Input: part model. Units: mm. Frame: model coordinates. A direction names the side the tool comes from. Round coordinates to 2 decimals unless told otherwise and drop trailing zeros. Loops run counter-clockwise (first coordinate to the right, second up) from the corner with the lowest first, then second, coordinate; pieces in that order, holes last. Notation, with made-up numbers: (-12, 25.5) -> (8, 25.5) arc R13 cw to (8, 47.5) -> close; hole circle Ø11 at (0.25, 70). An arc over 180 degrees is marked (long way). Answer as a JSON object with one key per item and string values. Group by question number.
Item 1: Section query C-C on x = 5.5. Return loops of the section in (y, z).
Item 2: Set-up query: faces 5 (the flat face through (-12, 17, 4)), 6 (the flat face through (2, -27, -2)), 7 (the flat face through (9.5, -32, 4)), 8 (the flat face through (2.7, -23, -3.5)). Return all of +Z, -Z, +X, -X, +Y, -Y with unobstructed straight access to the full face (end or side cutting, diameter ignored); none if empty.
Item 3: Section query A-A on y = 6. Return loops of the section in (x, z).
Item 4: Section query B-B on z = 11.2. Return loops of the section in (x, y).
Item 5: Pin query (flat end, axial travel): pin 1 (15.5 mm diameter, centred on x = 7.5, y = -9.5, fed in from -Z); pin 2 (7.5 mm diameter, centred on x = -5, z = 7, fed in from +Y); pin 3 (0.5 mm diameter, centred on x = -2.5, z = 1, fed in from -Y); pin 4 (3 mm diameter, centred on x = -8, z = 11.2, fed in from +Y). Return the tip coordinate at first contact, or that it passes through.
Item 6: Section query D-D on x = 10.5. Return loops of the section in (y, z).
Item 7: Draft query along Z for faces 1 (the flat face through (3, -30, 9)), 2 (the flat face through (3, -24, -4)), 3 (the flat face through (-14, -17, 7)), 4 (the flat face through (-11, 15, 7)). Return one class per face: released by +Z, released by -Z, zero draft, split by the parting line, or undercut.
Item 8: Material intervals for line 1 (Y direction, x = -10, z = 5.75); line 2 (X direction, y = 15.05, z = 4.5); line 3 (Z direction, x = 13, y = -31.2), sorted ascending. Write a range as [from, to].
from build123d import *

# Parameters (mm, degrees)
SKETCH_1_W           = 35
SKETCH_1_H           = 53
EXTRUDE_1_DEPTH      = 2
SKETCH_2_W           = 2
SKETCH_2_H           = 53
EXTRUDE_2_DEPTH      = 13.2
SKETCH_3_W           = 31
SKETCH_3_H           = 3
EXTRUDE_3_DEPTH      = 7.2
SKETCH_4_W           = 31
SKETCH_4_H           = 3
EXTRUDE_4_DEPTH      = 13.2
CUT_EXTRUDE_1_REACH  = 57.956
SKETCH_5_R           = 1.25
SKETCH_7_W           = 31
SKETCH_7_H           = 3
CUT_EXTRUDE_2_DEPTH  = 2.2
SKETCH_8_W           = 31
SKETCH_8_H           = 3
CUT_EXTRUDE_3_DEPTH  = 2
SKETCH_10_W          = 11
SKETCH_10_H          = 3
CUT_EXTRUDE_4_DEPTH  = 4
CUT_EXTRUDE_START    = -3
SKETCH_9_R           = 1.25
CUT_EXTRUDE_5_DEPTH  = 3
SKETCH_14_W          = 31
SKETCH_14_H          = 3
CUT_EXTRUDE_8_DEPTH  = 5
SKETCH_15_W          = 35
SKETCH_15_H          = 53
SKETCH_15_W_2        = 26
SKETCH_15_H_2        = 36
EXTRUDE_5_DEPTH      = 1
SKETCH_15_3_W        = 26
SKETCH_15_3_H        = 36
CUT_EXTRUDE_9_DEPTH  = 2
SKETCH_15_4_W        = 35
SKETCH_15_4_H        = 53
SKETCH_15_4_W_2      = 26
SKETCH_15_4_H_2      = 36
EXTRUDE_6_DEPTH      = 1
SKETCH_14_2_W        = 31
SKETCH_14_2_H        = 3
CUT_EXTRUDE_10_DEPTH = 7.2
SKETCH_21_W          = 31
SKETCH_21_H          = 3
CUT_EXTRUDE_11_DEPTH = 4
SKETCH_9_6_W         = 31
SKETCH_9_6_H         = 4
SKETCH_9_6_R         = 1.25
EXTRUDE_8_DEPTH      = 3
SKETCH_9_7_W         = 31
SKETCH_9_7_H         = 4
SKETCH_9_7_R         = 1.25
CUT_EXTRUDE_12_DEPTH = 3
SKETCH_23_W          = 31
SKETCH_23_H          = 3
EXTRUDE_9_DEPTH      = 2
SKETCH_24_W          = 31
SKETCH_24_H          = 3
CUT_EXTRUDE_13_DEPTH = 7.2
SKETCH_25_R          = 1.2
CUT_EXTRUDE_14_DEPTH = 3
SKETCH_15_5_W        = 35
SKETCH_15_5_H        = 53
SKETCH_15_5_W_2      = 26
SKETCH_15_5_H_2      = 36
EXTRUDE_10_DEPTH     = 2
SKETCH_28_W          = 31
SKETCH_28_H          = 2.1
CUT_EXTRUDE_15_DEPTH = 47
SKETCH_21_2_W        = 31
SKETCH_21_2_H        = 3
CUT_EXTRUDE_16_DEPTH = 6
SKETCH_12_W          = 2
SKETCH_12_H          = 10
CUT_EXTRUDE_17_DEPTH = 13.2
SKETCH_12_2_W        = 2
SKETCH_12_2_H        = 10
EXTRUDE_11_DEPTH     = 8.2
SKETCH_33_W          = 14
SKETCH_33_H          = 5
CUT_EXTRUDE_18_DEPTH = 3
SKETCH_34_W          = 21
SKETCH_34_H          = 3
CUT_EXTRUDE_19_DEPTH = 5
CUT_EXTRUDE_20_DEPTH = 0.1
CUT_EXTRUDE_21_DEPTH = 0.1
SKETCH_38_W          = 31
SKETCH_38_H          = 47
SKETCH_38_W_2        = 26
SKETCH_38_H_2        = 36
EXTRUDE_12_DEPTH     = 2
SKETCH_39_W          = 26
SKETCH_39_H          = 36
CUT_EXTRUDE_22_DEPTH = 2
SKETCH_40_W          = 35
SKETCH_40_H          = 53
SKETCH_40_W_2        = 26
SKETCH_40_H_2        = 36
EXTRUDE_13_DEPTH     = 2
SKETCH_41_W          = 31
SKETCH_41_H          = 47
SKETCH_41_W_2        = 26
SKETCH_41_H_2        = 36
CUT_EXTRUDE_23_DEPTH = 2
EXTRUDE_14_DEPTH     = 1.8


with BuildPart() as part:
    # 草图1 → 凸台-拉伸1 (new body)
    with BuildSketch(Plane.XY):
        with Locations((2.5, -6.5)):
            Rectangle(SKETCH_1_W, SKETCH_1_H)
    extrude(amount=EXTRUDE_1_DEPTH)

    # 草图2 → 凸台-拉伸2 (add)
    with BuildSketch(Plane.XY.offset(2)):
        with Locations((-14, -6.5)):
            Rectangle(SKETCH_2_W, SKETCH_2_H)
        with Locations((19, -6.5)):
            Rectangle(SKETCH_2_W, SKETCH_2_H)
    extrude(amount=EXTRUDE_2_DEPTH)

    # 草图3 → 凸台-拉伸3 (add)
    with BuildSketch(Plane.XY.offset(2)):
        with Locations((2.5, 18.5)):
            Rectangle(SKETCH_3_W, SKETCH_3_H)
        with Locations((2.5, -31.5)):
            Rectangle(SKETCH_3_W, SKETCH_3_H)
    extrude(amount=EXTRUDE_3_DEPTH)

    # 草图4 → 凸台-拉伸4 (add)
    with BuildSketch(Plane.XY.offset(2)):
        with Locations((2.5, 15.5)):
            Rectangle(SKETCH_4_W, SKETCH_4_H)
        with Locations((2.5, -28.5)):
            Rectangle(SKETCH_4_W, SKETCH_4_H)
    extrude(amount=EXTRUDE_4_DEPTH)

    # 草图5 → 切除-拉伸1 (cut, up to next)
    with BuildSketch(Plane(origin=(0, 17, 0), x_dir=(1, 0, 0), z_dir=(0, 1, 0)), mode=Mode.PRIVATE) as cut_extrude_1_sk1:
        with Locations(Location((-8, -11.2, 0), (0, 0, 270))):
            Circle(SKETCH_5_R)
    cut_extrude_1_tool1 = extrude(cut_extrude_1_sk1.sketch, amount=-CUT_EXTRUDE_1_REACH, mode=Mode.PRIVATE) & part.part
    # 草图5 → 切除-拉伸1 (cut, up to next)
    with BuildSketch(Plane(origin=(0, 17, 0), x_dir=(1, 0, 0), z_dir=(0, 1, 0)), mode=Mode.PRIVATE) as cut_extrude_1_sk2:
        with Locations(Location((2.5, -11.2, 0), (0, 0, 270))):
            Circle(SKETCH_5_R)
    cut_extrude_1_tool2 = extrude(cut_extrude_1_sk2.sketch, amount=-CUT_EXTRUDE_1_REACH, mode=Mode.PRIVATE) & part.part
    # 草图5 → 切除-拉伸1 (cut, up to next)
    with BuildSketch(Plane(origin=(0, 17, 0), x_dir=(1, 0, 0), z_dir=(0, 1, 0)), mode=Mode.PRIVATE) as cut_extrude_1_sk3:
        with Locations(Location((13, -11.2, 0), (0, 0, 270))):
            Circle(SKETCH_5_R)
    cut_extrude_1_tool3 = extrude(cut_extrude_1_sk3.sketch, amount=-CUT_EXTRUDE_1_REACH, mode=Mode.PRIVATE) & part.part
    add(cut_extrude_1_tool1.solids().sort_by_distance((-8, 17, 11.2))[0], mode=Mode.SUBTRACT)
    add(cut_extrude_1_tool2.solids().sort_by_distance((2.5, 17, 11.2))[0], mode=Mode.SUBTRACT)
    add(cut_extrude_1_tool3.solids().sort_by_distance((13, 17, 11.2))[0], mode=Mode.SUBTRACT)

    # 草图7 → 切除-拉伸2 (cut)
    with BuildSketch(Plane.XY.offset(15.2)):
        with Locations((2.5, 15.5)):
            Rectangle(SKETCH_7_W, SKETCH_7_H)
    extrude(amount=-CUT_EXTRUDE_2_DEPTH, mode=Mode.SUBTRACT)

    # 草图8 → 切除-拉伸3 (cut)
    with BuildSketch(Plane.XY.offset(15.2)):
        with Locations((2.5, -28.5)):
            Rectangle(SKETCH_8_W, SKETCH_8_H)
    extrude(amount=-CUT_EXTRUDE_3_DEPTH, mode=Mode.SUBTRACT)

    # 草图10 → 切除-拉伸4 (cut)
    with BuildSketch(Plane.XY.offset(13.2)):
        with Locations((2.5, -28.5)):
            Rectangle(SKETCH_10_W, SKETCH_10_H)
    extrude(amount=-CUT_EXTRUDE_4_DEPTH, mode=Mode.SUBTRACT)

    # 草图9 → 切除-拉伸5 (cut)
    with BuildSketch(Plane.XZ.offset(30).offset(CUT_EXTRUDE_START)):
        with Locations(Location((-8, 11.2, 0), (0, 0, 90))):
            Circle(SKETCH_9_R)
        with Locations(Location((13, 11.2, 0), (0, 0, 90))):
            Circle(SKETCH_9_R)
    extrude(amount=CUT_EXTRUDE_5_DEPTH, mode=Mode.SUBTRACT)

    # 草图14 → 切除-拉伸8 (cut)
    with BuildSketch(Plane.XY.offset(9.2)):
        with Locations((2.5, 18.5)):
            Rectangle(SKETCH_14_W, SKETCH_14_H)
    extrude(amount=-CUT_EXTRUDE_8_DEPTH, mode=Mode.SUBTRACT)

    # 草图15 → 凸台-拉伸5 (add)
    with BuildSketch(Plane(origin=(0, 0, 0), x_dir=(-1, 0, 0), z_dir=(0, 0, -1))):
        with Locations((-2.5, -6.5)):
            Rectangle(SKETCH_15_W, SKETCH_15_H)
        with Locations((-2.5, -5)):
            Rectangle(SKETCH_15_W_2, SKETCH_15_H_2, mode=Mode.SUBTRACT)
    extrude(amount=EXTRUDE_5_DEPTH)

    # 草图15<3> → 切除-拉伸9 (cut)
    with BuildSketch(Plane(origin=(0, 0, 0), x_dir=(-1, 0, 0), z_dir=(0, 0, -1))):
        with Locations((-2.5, -5)):
            Rectangle(SKETCH_15_3_W, SKETCH_15_3_H)
    extrude(amount=-CUT_EXTRUDE_9_DEPTH, mode=Mode.SUBTRACT)

    # 草图15<4> → 凸台-拉伸6 (add)
    with BuildSketch(Plane(origin=(0, 0, 0), x_dir=(-1, 0, 0), z_dir=(0, 0, -1))):
        with Locations((-2.5, -6.5)):
            Rectangle(SKETCH_15_4_W, SKETCH_15_4_H)
        with Locations((-2.5, -5)):
            Rectangle(SKETCH_15_4_W_2, SKETCH_15_4_H_2, mode=Mode.SUBTRACT)
    extrude(amount=EXTRUDE_6_DEPTH)

    # 草图14<2> → 切除-拉伸10 (cut)
    with BuildSketch(Plane.XY.offset(9.2)):
        with Locations((2.5, 18.5)):
            Rectangle(SKETCH_14_2_W, SKETCH_14_2_H)
    extrude(amount=-CUT_EXTRUDE_10_DEPTH, mode=Mode.SUBTRACT)

    # 草图21 → 切除-拉伸11 (cut)
    with BuildSketch(Plane.XY.offset(13)):
        with Locations((2.5, 15.5)):
            Rectangle(SKETCH_21_W, SKETCH_21_H)
    extrude(amount=-CUT_EXTRUDE_11_DEPTH, mode=Mode.SUBTRACT)

    # 草图9<6> → 凸台-拉伸8 (add)
    with BuildSketch(Plane.XZ.offset(30)):
        with Locations((2.5, 11.2)):
            Rectangle(SKETCH_9_6_W, SKETCH_9_6_H)
        with Locations((13, 11.2)):
            Circle(SKETCH_9_6_R, mode=Mode.SUBTRACT)
        with Locations((-8, 11.2)):
            Circle(SKETCH_9_6_R, mode=Mode.SUBTRACT)
    extrude(amount=EXTRUDE_8_DEPTH)

    # 草图9<7> → 切除-拉伸12 (cut)
    with BuildSketch(Plane.XZ.offset(30).offset(CUT_EXTRUDE_START)):
        with Locations((2.5, 11.2)):
            Rectangle(SKETCH_9_7_W, SKETCH_9_7_H)
        with Locations(Location((13, 11.2, 0), (0, 0, 270))):
            Circle(SKETCH_9_7_R, mode=Mode.SUBTRACT)
        with Locations(Location((-8, 11.2, 0), (0, 0, 270))):
            Circle(SKETCH_9_7_R, mode=Mode.SUBTRACT)
    extrude(amount=CUT_EXTRUDE_12_DEPTH, mode=Mode.SUBTRACT)

    # 草图23 → 凸台-拉伸9 (add)
    with BuildSketch(Plane.XY.offset(13.2)):
        with Locations((2.5, -31.5)):
            Rectangle(SKETCH_23_W, SKETCH_23_H)
    extrude(amount=EXTRUDE_9_DEPTH)

    # 草图24 → 切除-拉伸13 (cut)
    with BuildSketch(Plane.XY.offset(9.2)):
        with Locations((2.5, -28.5)):
            Rectangle(SKETCH_24_W, SKETCH_24_H)
    extrude(amount=-CUT_EXTRUDE_13_DEPTH, mode=Mode.SUBTRACT)

    # 草图25 → 切除-拉伸14 (cut)
    with BuildSketch(Plane(origin=(0, 17, 0), x_dir=(1, 0, 0), z_dir=(0, 1, 0))):
        with Locations(Location((-10.5, -4.5, 0), (0, 0, 270))):
            Circle(SKETCH_25_R)
        with Locations(Location((15.5, -4.5, 0), (0, 0, 270))):
            Circle(SKETCH_25_R)
    extrude(amount=-CUT_EXTRUDE_14_DEPTH, mode=Mode.SUBTRACT)

    # 草图15<5> → 凸台-拉伸10 (add)
    with BuildSketch(Plane(origin=(0, 0, 0), x_dir=(-1, 0, 0), z_dir=(0, 0, -1))):
        with Locations((-2.5, -6.5)):
            Rectangle(SKETCH_15_5_W, SKETCH_15_5_H)
        with Locations((-2.5, -5)):
            Rectangle(SKETCH_15_5_W_2, SKETCH_15_5_H_2, mode=Mode.SUBTRACT)
    extrude(amount=EXTRUDE_10_DEPTH)

    # 草图28 → 切除-拉伸15 (cut)
    with BuildSketch(Plane(origin=(0, 20, 0), x_dir=(1, 0, 0), z_dir=(0, 1, 0))):
        with Locations((2.5, -0.05)):
            Rectangle(SKETCH_28_W, SKETCH_28_H)
    extrude(amount=-CUT_EXTRUDE_15_DEPTH, mode=Mode.SUBTRACT)

    # 草图21<2> → 切除-拉伸16 (cut)
    with BuildSketch(Plane.XY.offset(13)):
        with Locations((2.5, 15.5)):
            Rectangle(SKETCH_21_2_W, SKETCH_21_2_H)
    extrude(amount=-CUT_EXTRUDE_16_DEPTH, mode=Mode.SUBTRACT)

    # 草图12 → 切除-拉伸17 (cut)
    with BuildSketch(Plane.XY.offset(15.2)):
        with Locations((-14, -17.5)):
            Rectangle(SKETCH_12_W, SKETCH_12_H)
    extrude(amount=-CUT_EXTRUDE_17_DEPTH, mode=Mode.SUBTRACT)

    # 草图12<2> → 凸台-拉伸11 (add)
    with BuildSketch(Plane.XY.offset(15.2)):
        with Locations((-14, -17.5)):
            Rectangle(SKETCH_12_2_W, SKETCH_12_2_H)
    extrude(amount=-EXTRUDE_11_DEPTH)

    # 草图33 → 切除-拉伸18 (cut)
    with BuildSketch(Plane.XZ.offset(33)):
        with Locations((2.5, 4.5)):
            Rectangle(SKETCH_33_W, SKETCH_33_H)
    extrude(amount=-CUT_EXTRUDE_18_DEPTH, mode=Mode.SUBTRACT)

    # 草图34 → 切除-拉伸19 (cut)
    with BuildSketch(Plane.XY.offset(7)):
        with Locations((2.5, 15.5)):
            Rectangle(SKETCH_34_W, SKETCH_34_H)
    extrude(amount=-CUT_EXTRUDE_19_DEPTH, mode=Mode.SUBTRACT)

    # 草图35 → 切除-拉伸20 (cut)
    with BuildSketch(Plane.ZY.offset(-18)):
        Polygon((2, 20), (2, 17), (7, 17), (7, 14), (2, 14), (2, -30), (15.2, -30), (15.2, 20), align=None)
    extrude(amount=-CUT_EXTRUDE_20_DEPTH, mode=Mode.SUBTRACT)

    # 草图36 → 切除-拉伸21 (cut)
    with BuildSketch(Plane(origin=(-13, 0, 0), x_dir=(0, 0, -1), z_dir=(1, 0, 0))):
        Polygon((-15.2, -30), (-2, -30), (-2, -22.5), (-7, -22.5), (-7, -12.5), (-2, -12.5), (-2, 14), (-7, 14), (-7, 17), (-2, 17), (-2, 20), (-15.2, 20), align=None)
    extrude(amount=-CUT_EXTRUDE_21_DEPTH, mode=Mode.SUBTRACT)

    # 草图38 → 凸台-拉伸12 (add)
    with BuildSketch(Plane(origin=(0, 0, 1.1), x_dir=(-1, 0, 0), z_dir=(0, 0, -1))):
        with Locations((-2.5, -3.5)):
            Rectangle(SKETCH_38_W, SKETCH_38_H)
        with Locations((-2.5, -5)):
            Rectangle(SKETCH_38_W_2, SKETCH_38_H_2, mode=Mode.SUBTRACT)
    extrude(amount=EXTRUDE_12_DEPTH)

    # 草图39 → 切除-拉伸22 (cut)
    with BuildSketch(Plane.XY.offset(2)):
        Polygon((-15, -12.5), (-15, -22.5), (-13.1, -22.5), (-13.1, -30), (-4.5, -30), (-4.5, -33), (9.5, -33), (9.5, -30), (18.1, -30), (18.1, 14), (13, 14), (13, 17), (18.1, 17), (18.1, 20), (-13.1, 20), (-13.1, 17), (-8, 17), (-8, 14), (-13.1, 14), (-13.1, -12.5), align=None)
        with Locations((2.5, -5)):
            Rectangle(SKETCH_39_W, SKETCH_39_H, mode=Mode.SUBTRACT)
    extrude(amount=-CUT_EXTRUDE_22_DEPTH, mode=Mode.SUBTRACT)

    # 草图40 → 凸台-拉伸13 (add)
    with BuildSketch(Plane(origin=(0, 0, -2), x_dir=(-1, 0, 0), z_dir=(0, 0, -1))):
        with Locations((-2.5, -6.5)):
            Rectangle(SKETCH_40_W, SKETCH_40_H)
        with Locations((-2.5, -5)):
            Rectangle(SKETCH_40_W_2, SKETCH_40_H_2, mode=Mode.SUBTRACT)
    extrude(amount=EXTRUDE_13_DEPTH)

    # 草图41 → 切除-拉伸23 (cut)
    with BuildSketch(Plane.XY.offset(-1)):
        with Locations((2.5, -3.5)):
            Rectangle(SKETCH_41_W, SKETCH_41_H)
        with Locations((2.5, -5)):
            Rectangle(SKETCH_41_W_2, SKETCH_41_H_2, mode=Mode.SUBTRACT)
    extrude(amount=-CUT_EXTRUDE_23_DEPTH, mode=Mode.SUBTRACT)

    # 草图42 → 凸台-拉伸14 (add)
    with BuildSketch(Plane.XY):
        Polygon((-8, 17), (13, 17), (18.1, 17), (18.1, 20), (-13.1, 20), (-13.1, 17), align=None)
    extrude(amount=EXTRUDE_14_DEPTH)


solid = part.part
Solved:
{
 "1": {"outline": "(-33, -4) -> (-23, -4) -> (-23, -3) -> (-27, -3) -> (-27, -0.9) -> (-23, -0.9) -> (-23, 0) -> (-33, 0) -> close; (-33, 7) -> (-30, 7) -> (-30, 15.2) -> (-33, 15.2) -> close; (13, -4) -> (20, -4) -> (20, -3) -> (13, -3) -> close; (13, -0.9) -> (20, -0.9) -> (20, 1.8) -> (17, 1.8) -> (17, 0) -> (13, 0) -> close"},
 "2": {"face 5": "+Z, +Y", "face 6": "+Y", "face 7": "-Y", "face 8": "+Z, -Z"},
 "3": {"outline": "(-15, -4) -> (-10.5, -4) -> (-10.5, -3) -> (-13, -3) -> (-13, -0.9) -> (-10.5, -0.9) -> (-10.5, 0) -> (-13.1, 0) -> (-13.1, 15.2) -> (-15, 15.2) -> close; (15.5, -4) -> (20, -4) -> (20, 15.2) -> (18.1, 15.2) -> (18.1, 0) -> (15.5, 0) -> (15.5, -0.9) -> (18, -0.9) -> (18, -3) -> (15.5, -3) -> close"},
 "4": {"outline": "(-15, -33) -> (-9.25, -33) -> (-9.25, -30) -> (-13.1, -30) -> (-13.1, 20) -> (-15, 20) -> close; (-6.75, -33) -> (11.75, -33) -> (11.75, -30) -> (-6.75, -30) -> close; (14.25, -33) -> (20, -33) -> (20, 20) -> (18.1, 20) -> (18.1, -30) -> (14.25, -30) -> close"},
 "5": {"pin 1": "through", "pin 2": "y = 17", "pin 3": "y = 17", "pin 4": "y = -30"},
 "6": {"outline": "(-33, -4) -> (-23, -4) -> (-23, -3) -> (-27, -3) -> (-27, -0.9) -> (-23, -0.9) -> (-23, 0) -> (-30, 0) -> (-30, 15.2) -> (-33, 15.2) -> close; (13, -4) -> (20, -4) -> (20, -3) -> (13, -3) -> close; (13, -0.9) -> (20, -0.9) -> (20, 1.8) -> (17, 1.8) -> (17, 0) -> (13, 0) -> close"},
 "7": {"face 1": "zero draft", "face 2": "released by -Z", "face 3": "undercut", "face 4": "released by +Z"},
 "8": {"line 1": "[-33, -30], [14, 17]", "line 2": "[-15, -11.7], [-9.3, -8], [13, 14.3], [16.7, 20]", "line 3": "[-4, 9.95], [12.45, 15.2]"}
}
